```python
from build123d import *

# Parameters (mm, degrees)
SKETCH3_R                 = 4
BOSS_EXTRUDE1_DEPTH       = 15
BOSS_EXTRUDE2_START       = 15
SKETCH3_3_R               = 5
BOSS_EXTRUDE2_DEPTH       = 5
BOSS_EXTRUDE3_START       = 20
BOSS_EXTRUDE3_DEPTH       = 2.5
CUT_EXTRUDE1_DEPTH        = 15
GRUB_START                = -4.0000001
GRUB_SCREW_HOLE_OUTLINE_R = 1.5
GRUB_SCREW_HOLE_DEPTH     = 3.0000001


# Read off the part's stored shape, not the designer's step: Grub Screw Hole
with BuildPart() as part:
    # Sketch3 → Boss-Extrude1 (new body)
    with BuildSketch(Plane(origin=(0, 0, 0), x_dir=(1, 0, 0), z_dir=(0, 1, 0))):
        with Locations(Location((0, 0, 0), (0, 0, 270))):
            Circle(SKETCH3_R)
    extrude(amount=BOSS_EXTRUDE1_DEPTH)

    # Sketch3<3> → Boss-Extrude2 (add)
    with BuildSketch(Plane(origin=(0, 0, 0), x_dir=(1, 0, 0), z_dir=(0, 1, 0)).offset(BOSS_EXTRUDE2_START)):
        with Locations(Location((0, 0, 0), (0, 0, 270))):
            Circle(SKETCH3_3_R)
    extrude(amount=BOSS_EXTRUDE2_DEPTH)

    # Sketch3<5> → Boss-Extrude3 (add)
    with BuildSketch(Plane(origin=(0, 0, 0), x_dir=(1, 0, 0), z_dir=(0, 1, 0)).offset(BOSS_EXTRUDE3_START)):
        with BuildLine():
            Line((-5, -8.5), (-5, 8.5))
            ThreePointArc((-5, 8.5), (0, 13.5), (5, 8.5))
            Line((5, 8.5), (5, -8.5))
            ThreePointArc((5, -8.5), (0, -13.5), (-5, -8.5))
        make_face()
    extrude(amount=-BOSS_EXTRUDE3_DEPTH)

    # Sketch5 → Cut-Extrude1 (cut)
    with BuildSketch(Plane(origin=(0, 0, 0), x_dir=(1, 0, 0), z_dir=(0, 1, 0))):
        with BuildLine():
            ThreePointArc((2, 0), (1, 1.732050808), (-1, 1.732050808))
            Line((-1, 1.732050808), (-1, -1.732050808))
            ThreePointArc((-1, -1.732050808), (1, -1.732050808), (2, 0))
        make_face()
    extrude(amount=CUT_EXTRUDE1_DEPTH, mode=Mode.SUBTRACT)

    # Grub Screw Hole outline → Grub Screw Hole (cut)
    with BuildSketch(Plane(origin=(0, 0, 0), x_dir=(0, 0, -1), z_dir=(1, 0, 0)).offset(GRUB_START)):
        with Locations((0, 5)):
            Circle(GRUB_SCREW_HOLE_OUTLINE_R)
    extrude(amount=GRUB_SCREW_HOLE_DEPTH, mode=Mode.SUBTRACT)


solid = part.part
```
Input: part model. Units: mm. Frame: model coordinates. A direction names the side the tool comes from. Coordinates: 2 decimals unless noted, no trailing zeros. Loops run counter-clockwise (first coordinate to the right, second up) from the corner with the lowest first, then second, coordinate; pieces in that order, holes last. Notation, with made-up numbers: M -17.5,20.5 L -6.5,20.5 A13 cw -6.5,41.5 Z; hole C 31,-4 d9. An arc over 180 degrees is marked long. Use a Markdown table: item, result. Add a question column.
1) Section B-B, the plane y = 8. Return the cut outline in (x, z), plus the area to 3 significant figures.
2) Set-up query: faces 4 (the cylindrical face through (3.966, 7.395, -0.521)), 5 (the flat face through (5, 19, 0)). Return all of +Z, -Z, +X, -X, +Y, -Y with unobstructed straight access to the full face (end or side cutting, diameter ignored); none if empty.
3) Pin query (flat end, axial travel): P1, Ø2.5, axis at y = 5, z = 0, coming from the +X side; P2, Ø10, axis at y = 10.5, z = -1, coming from the -X side; P3, Ø1, axis at x = -1, z = 6.5, coming from the -Y side; P4, Ø0.9, axis at x = 0.5, z = 1, coming from the -Y side. Return the tip coordinate at first contact, or that it passes through.
4) Section A-A, the plane x = 0. Return the cut outline in (y, z), plus the area to 4 significant figures.
5) Section D-D, the plane x = -2.25. Return the cut outline in (y, z), plus the area to 3 significant figures.
6) Draft query along Z for faces 1 (the flat face through (0, 20, 0)), 2 (the cylindrical face through (-2.52, 5.45, -1.43)), 3 (the cylindrical face through (0.1, 18.8, 13.5)). Return one class per face: +Z half, -Z half, draft (parallel to the pull), parting line (faces both ways), or undercut.
7) Line query: L1, parallel to Y at x = -2.65, z = 0; L2, parallel to Y at x = -1.75, z = 12.5; L3, parallel to Z at x = -3.2, y = 5. Output: solid intervals per line, ascending. Write a range as from..to.
8) Section C-C, the plane z = -0.75. Return the cut outline in (x, y).
Answer below:
| question | item | result |
|---|---|---|
| 1 | outline | C 0,0 d8; hole M -1,-1.73 A2 ccw long -1,1.73 Z |
| 1 | area | 40.2 mm2 |
| 2 | face 4 | -Y |
| 2 | face 5 | +Z, -Z, +X, +Y, -Y |
| 3 | P1 | x = 4 |
| 3 | P2 | x = -5 |
| 3 | P3 | y = 17.5 |
| 3 | P4 | y = 15 |
| 4 | outline | M 0,-4 L 15,-4 L 15,-5 L 17.5,-5 L 17.5,-13.5 L 20,-13.5 L 20,13.5 L 17.5,13.5 L 17.5,5 L 15,5 L 15,4 L 0,4 L 0,2 L 15,2 L 15,-2 L 0,-2 Z |
| 4 | area | 152.5 mm2 |
| 5 | outline | M 0,-3.31 L 15,-3.31 L 15,-4.47 L 17.5,-4.47 L 17.5,-12.97 L 20,-12.97 L 20,12.97 L 17.5,12.97 L 17.5,4.47 L 15,4.47 L 15,3.31 L 0,3.31 Z; hole C 5,0 d3 |
| 5 | area | 179 mm2 |
| 6 | face 1 | draft |
| 6 | face 2 | undercut |
| 6 | face 3 | +Z half |
| 7 | L1 | 0..3.5, 6.5..20 |
| 7 | L2 | 17.5..20 |
| 7 | L3 | -2.4..-1.5, 1.5..2.4 |
| 8 | outline | M -5,17.5 L -4.94,17.5 L -4.94,15 L -3.93,15 L -3.93,6.3 L -1,6.3 L -1,15 L 1.85,15 L 1.85,0 L 3.93,0 L 3.93,15 L 4.94,15 L 4.94,17.5 L 5,17.5 L 5,20 L -5,20 Z; M -3.93,0 L -1,0 L -1,3.7 L -3.93,3.7 Z |
